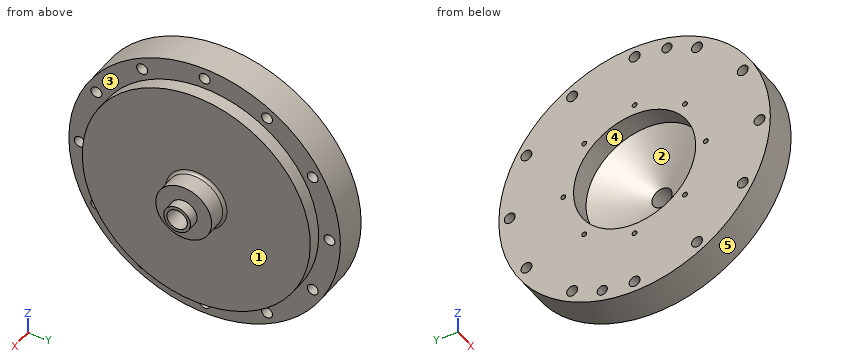
```python
from build123d import *

# Parameters (mm, degrees)
SKETCH3_R                 = 4.7625
OXIDIZER_INLET_HOLE_DEPTH = 37.83
FLANGE_HOLES_D            = 5.1054
FLANGE_HOLES_DEPTH        = 22.225
DOWEL_HOLES_D             = 4.7625
DOWEL_HOLES_DEPTH         = 6.35
DOWEL_HOLES_TIP           = 1.430799349
SKETCH12_R                = 28.575
CUT_EXTRUDE2_DEPTH        = 9.525
SKETCH16_R                = 28.575
SKETCH17_R                = 4.7625
CIRPATTERN1_COUNT         = 8
FILLET1_R                 = 1.27
SKETCH25_OUTSIDE_W        = 165.668
SKETCH25_OUTSIDE_H        = 165.668
SKETCH25_OUTSIDE_R        = 53.34
CUT_EXTRUDE3_DEPTH        = 6.35


with BuildPart() as part:
    # Sketch2 → Main Structure (revolve)
    with BuildSketch(Plane.XY):
        Polygon((41.355, 13.081), (41.355, 6.2484), (46.355, 6.2484), (46.355, 0), (9.525, 0), (9.525, 63.5), (31.75, 63.5), (31.75, 13.081), align=None)
    revolve(axis=Axis((9.525, 0, 0), (1, 0, 0)))

    # Sketch3 → Oxidizer Inlet Hole (cut, through all)
    with BuildSketch(Plane(origin=(46.355, 0, 0), x_dir=(0, 0, -1), z_dir=(1, 0, 0))):
        Circle(SKETCH3_R)
    extrude(amount=-OXIDIZER_INLET_HOLE_DEPTH, mode=Mode.SUBTRACT)

    # Flange Holes
    with Locations(Plane(origin=(31.75, 0, 0), x_dir=(0, 0, 1), z_dir=(1, 0, 0))):
        with Locations((0, 58.42), (-29.21, 50.593204089), (-50.593204089, 29.21), (-58.42, 0), (-50.593204089, -29.21), (-29.21, -50.593204089), (0, -58.42), (29.21, -50.593204089), (50.593204089, -29.21), (58.42, 0), (50.593204089, 29.21), (29.21, 50.593204089)):
            Hole(FLANGE_HOLES_D / 2, depth=FLANGE_HOLES_DEPTH)

    # Dowel Holes
    with Locations(Plane.ZY.offset(-9.525)):
        with Locations((56.429386772, -15.120208615), (-56.429386772, 15.120208615)):
            Hole(DOWEL_HOLES_D / 2, depth=DOWEL_HOLES_DEPTH)
            with Locations((0, 0, -(DOWEL_HOLES_DEPTH + DOWEL_HOLES_TIP / 2))):  # 118° drill point
                Cone(0, DOWEL_HOLES_D / 2, DOWEL_HOLES_TIP, mode=Mode.SUBTRACT)

    # Sketch12 → Cut-Extrude2 (cut)
    with BuildSketch(Plane.ZY.offset(-9.525)):
        Circle(SKETCH12_R)
    extrude(amount=-CUT_EXTRUDE2_DEPTH, mode=Mode.SUBTRACT)

    # Sketch16 → Internal Flow Path Loft Cut section 0
    with BuildSketch(Plane.ZY.offset(-19.05)):
        Circle(SKETCH16_R)
    # Sketch17 → Internal Flow Path Loft Cut section 1
    with BuildSketch(Plane.ZY.offset(-30.48)):
        Circle(SKETCH17_R)
    loft(mode=Mode.SUBTRACT)

    # Sketch20 → #4-40 Tapped Hole1 (revolve, cut)
    with BuildSketch(Plane(origin=(9.525, 0, 33.3375), x_dir=(0, 0, 1), z_dir=(0, 1, 0))):
        Polygon((0, 0), (0, 13.887152758), (1.1303, 13.208), (1.1303, 0), align=None)
    f_4_40_tapped_hole1 = revolve(axis=Axis((3.175, 0, 33.3375), (1, 0, 0)), mode=Mode.SUBTRACT)

    # CirPattern1: #4-40 Tapped Hole1 ×8 about axis
    cirpattern1_axis = Axis((0, 0, 0), (1, 0, 0))
    for i in range(1, CIRPATTERN1_COUNT):
        add(f_4_40_tapped_hole1.rotate(cirpattern1_axis, i * 360 / CIRPATTERN1_COUNT), mode=Mode.SUBTRACT)

    # Fillet1
    fillet1_edges = [part.edges().sort_by_distance(p)[0] for p in [
        (31.75, -13.081, 0),
    ]]
    fillet(fillet1_edges, radius=FILLET1_R)

    # Sketch25 outside → Cut-Extrude3 (cut)
    with BuildSketch(Plane(origin=(31.75, 0, 0), x_dir=(0, 0, -1), z_dir=(1, 0, 0))):
        Rectangle(SKETCH25_OUTSIDE_W, SKETCH25_OUTSIDE_H)
        Circle(SKETCH25_OUTSIDE_R, mode=Mode.SUBTRACT)
    extrude(amount=-CUT_EXTRUDE3_DEPTH, mode=Mode.SUBTRACT)


solid = part.part
```
Geometry check sheet. Reference: the model listing, model coordinates, mm. Face numbers are marked on the shaded views. A direction names the side the tool comes from. Give positions to 0.01 mm unless a question says otherwise; leave off trailing zeros. Write each loop counter-clockwise with the first axis right and the second up, starting at its lowest first coordinate (ties: lowest second). Pieces come first, ordered by that corner, then holes.
1) Section check C-C, the plane y = 36.5. Record the boundary of the cut face in (x, z) (3 decimals), and give its area (3 significant figures).
2) Section check A-A, the plane y = 58.42. Record the boundary of the cut face in (x, z) (3 decimals).
3) Material ranges on L1, parallel to Y at x = 22, z = -49.5; L2, parallel to Z at x = 12, y = 50.5; L3, parallel to X at y = -8, z = -30 (3 decimals), recorded low to high.
4) Access from +Z, -Z, +X, -X, +Y, -Y to the whole of each face (thin tool, end or side, straight path). Record for the marked faces 1 and 2.
5) Section check B-B, the plane x = 36.5. Record the boundary of the cut face in (y, z) (1 decimal).
6) Gauge pin test, flat ends, axial feed: pin 1 (12 mm diameter, centred on x = 37.5, y = -26.5, fed in from -Z); pin 2 (2 mm diameter, centred on x = 23.5, z = -8, fed in from +Y); pin 3 (2 mm diameter, centred on x = 26, z = 9, fed in from -Y); pin 4 (4.5 mm diameter, centred on y = 58.42, z = 0, fed in from +X). Record the tip position at first contact, or that the pin passes through.
7) Release check for a two-part mould opening along Z. For the marked faces 3, 4 and 5 record: pulls with the +Z half, pulls with the -Z half, needs draft (parallel to the pull), parting line crosses it, or undercut.
Computed:
1. outline: (9.525, -51.962) - (25.4, -51.962) - (25.4, -38.896) - (31.75, -38.896) - (31.75, 38.896) - (25.4, 38.896) - (25.4, 51.962) - (9.525, 51.962) - close
1. area: 2,140 mm2
2. outline: (9.525, -24.887) - (25.4, -24.887) - (25.4, -2.553) - (9.525, -2.553) - close; (9.525, 2.553) - (25.4, 2.553) - (25.4, 24.887) - (9.525, 24.887) - close
3. L1: y = -39.77 to -31.52, -26.9 to 26.9, 31.52 to 39.77
3. L2: z = -38.5 to -31.76, -26.66 to 26.66, 31.76 to 38.5
3. L3: x = 9.525 to 31.75
4. face 1: +X
4. face 2: -X
5. outline: circle Ø26.2 at (0, 0); hole circle Ø9.5 at (0, 0)
6. pin 1: stops at z = -47.23
6. pin 2: stops at y = 63.11
6. pin 3: stops at y = -62.97
6. pin 4: passes through
7. face 3: needs draft
7. face 4: undercut
7. face 5: parting line crosses it
